The model under review builds one solid part; all positions refer to its coordinate system, in mm. Give positions to 0.01 mm unless a question says otherwise; leave off trailing zeros. Order: outer loops, then holes, each group sorted by start corner. A loop starts at its lowest first (then second) coordinate and runs counter-clockwise, first axis right, second up.
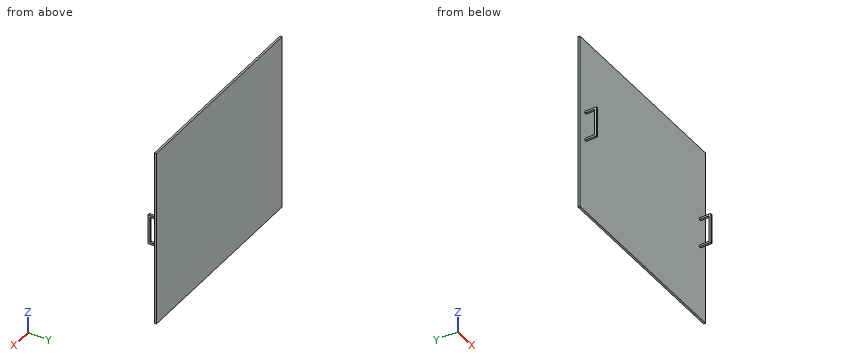
```python
from build123d import *

# Parameters (mm, degrees)
F0_W     = 643.89
F0_H     = 596.9
F1_DEPTH = 6.35
F2_W     = 6.35
F2_H     = 101.6
F3_DEPTH = 38.1
F4_W     = 31.75
F4_H     = 88.9
F5_DEPTH = 609.6


with BuildPart() as f1:
    # F0 (on Front) → F1 (new body)
    with BuildSketch(Plane.XZ):
        Rectangle(F0_W, F0_H)
    extrude(amount=F1_DEPTH)

    # F2 (on face) → F3 (join)
    with BuildSketch(Plane.XZ.offset(6.35)):
        with Locations((-293.37, 0)):
            Rectangle(F2_W, F2_H)
        with Locations((293.37, 0)):
            Rectangle(F2_W, F2_H)
    extrude(amount=F3_DEPTH)

    # F4 (on face) → F5 (cut)
    with BuildSketch(Plane(origin=(-296.545, 0, 0), x_dir=(0, -1, 0), z_dir=(-1, 0, 0))):
        with Locations((22.225, 0)):
            Rectangle(F4_W, F4_H)
    extrude(amount=-F5_DEPTH, mode=Mode.SUBTRACT)


solid = f1.part
```
1. Take a section at C-C (z = 256). Write out the cut boundary in (x, y) (3 decimals), and give its area (3 significant figures).
2. Take a section at A-A (z = -35). Write out the cut boundary in (x, y) (3 decimals), and give its area (3 significant figures).
3. Take a section at D-D (x = -248.5). Write out the cut boundary in (y, z).
4. Take a section at B-B (y = -16). Write out the cut boundary in (x, z) (3 decimals), and give its area (3 significant figures).
5. To check wall thickness, follow line 1 (X direction, y = -41.5, z = 8) (3 decimals); line 2 (Y direction, x = -283.5, z = 191). State the ranges of each line that lie inside material, in increasing order.
6. Insertion check: pin 1 (3 mm diameter, centred on x = -292, y = -17.5, fed in from +Z); pin 2 (3 mm diameter, centred on x = 295, y = -24.5, fed in from -Z); pin 3 (3 mm diameter, centred on x = 145.5, z = -3, fed in from -Y). Each pin has a flat end and moves straight along its axis. Give the tip position at first contact, or say it passes through.
Answer:
1. outline: (-321.945, -6.35) - (321.945, -6.35) - (321.945, 0) - (-321.945, 0) - close
1. area: 4,090 mm2
2. outline: (-321.945, -6.35) - (321.945, -6.35) - (321.945, 0) - (-321.945, 0) - close; (-296.545, -44.45) - (-290.195, -44.45) - (-290.195, -38.1) - (-296.545, -38.1) - close; (290.195, -44.45) - (296.545, -44.45) - (296.545, -38.1) - (290.195, -38.1) - close
2. area: 4,170 mm2
3. outline: (-6.35, -298.45) - (0, -298.45) - (0, 298.45) - (-6.35, 298.45) - close
4. outline: (-296.545, -50.8) - (-290.195, -50.8) - (-290.195, -44.45) - (-296.545, -44.45) - close; (-296.545, 44.45) - (-290.195, 44.45) - (-290.195, 50.8) - (-296.545, 50.8) - close; (290.195, -50.8) - (296.545, -50.8) - (296.545, -44.45) - (290.195, -44.45) - close; (290.195, 44.45) - (296.545, 44.45) - (296.545, 50.8) - (290.195, 50.8) - close
4. area: 161 mm2
5. line 1: x = -296.545 to -290.195, 290.195 to 296.545
5. line 2: y = -6.35 to 0
6. pin 1: stops at z = 50.8
6. pin 2: stops at z = -50.8
6. pin 3: stops at y = -6.35
